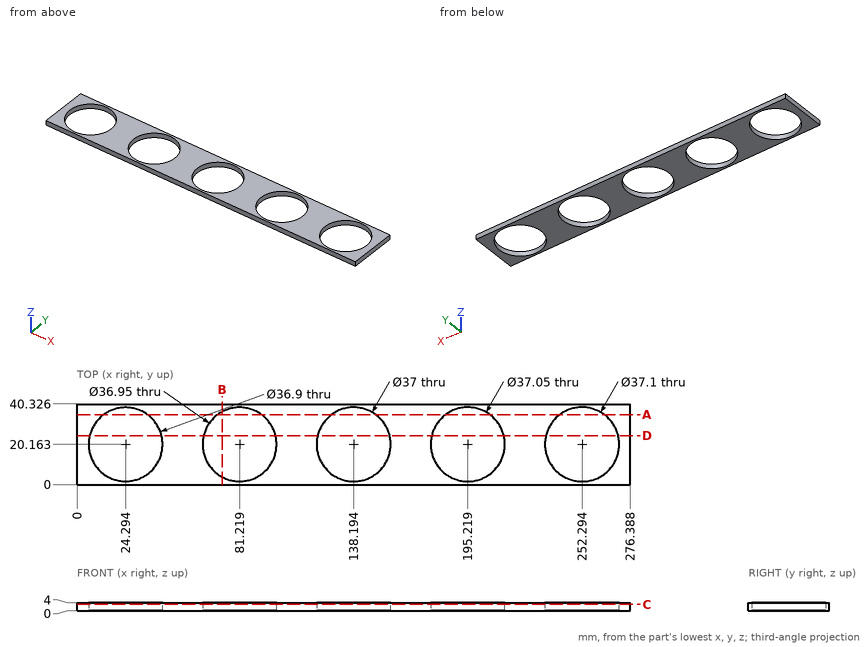
Could you check a few things on this drawing? It's one solid part, dimensions in mm from its lowest x, y, z. Round coordinates to 2 decimals unless told otherwise and drop trailing zeros. Order: outer loops, then holes, each group sorted by start corner. A loop starts at its lowest first (then second) coordinate and runs counter-clockwise, first axis right, second up. Notation, with made-up numbers: M 33.25,3 L 74.25,3 A33 cw 74.25,33 Z; hole C 36.25,57 d10. An arc over 180 degrees is marked long. Return JSON: item names as keys, results as strings. Group by question number.
1. If we section it at B-B on x = 72.5: List the corners of the cut face in (y, z) for me (1 decimal), then the cut area to 3 significant figures.
2. If we section it at A-A on y = 35: List the corners of the cut face in (x, z) for me.
3. If we section it at D-D on y = 24.5: List the corners of the cut face in (x, z) for me.
4. Please list where these lines run through material, in increasing order: probe 1 along X at (y, z) = (19, 2.8); probe 2 along X at (y, z) = (32, 0.8) (1 decimal); probe 3 along Y at (x, z) = (25, 2.65) (1 decimal).
5. If we section it at C-C on z = 3.2: State how many separate pieces and enclosed holes the cut face has, then the cut area to 3 significant figures.
Reply:
{
 "1": {"outline": "M 0,0 L 3.9,0 L 3.9,4 L 0,4 Z; M 36.5,0 L 40.3,0 L 40.3,4 L 36.5,4 Z", "area": "31.0 mm^2"},
 "2": {"outline": "M 0,0 L 13.33,0 L 13.33,4 L 0,4 Z; M 35.26,0 L 70.21,0 L 70.21,4 L 35.26,4 Z; M 92.23,0 L 127.14,0 L 127.14,4 L 92.23,4 Z; M 149.24,0 L 184.13,0 L 184.13,4 L 149.24,4 Z; M 206.31,0 L 241.16,0 L 241.16,4 L 206.31,4 Z; M 263.43,0 L 276.39,0 L 276.39,4 L 263.43,4 Z"},
 "3": {"outline": "M 0,0 L 6.36,0 L 6.36,4 L 0,4 Z; M 42.23,0 L 63.26,0 L 63.26,4 L 42.23,4 Z; M 99.18,0 L 120.21,0 L 120.21,4 L 99.18,4 Z; M 156.18,0 L 177.21,0 L 177.21,4 L 156.18,4 Z; M 213.23,0 L 234.26,0 L 234.26,4 L 213.23,4 Z; M 270.33,0 L 276.39,0 L 276.39,4 L 270.33,4 Z"},
 "4": {"probe 1": "0 to 5.88, 42.71 to 62.78, 99.66 to 119.73, 156.66 to 176.73, 213.71 to 233.78, 270.81 to 276.39", "probe 2": "0 to 10.1, 38.4 to 67, 95.4 to 124, 152.4 to 181, 209.5 to 238, 266.6 to 276.4", "probe 3": "0 to 1.7, 38.6 to 40.3"},
 "5": {"separate pieces": "1", "enclosed holes": "5", "area": "5,770 mm^2"}
}
